Job drawing, mm, ordinate dimensions from the low corner. One solid piece. A direction names the side the tool comes from. Coordinates: 2 decimals unless noted, no trailing zeros. Loops run counter-clockwise (first coordinate to the right, second up) from the corner with the lowest first, then second, coordinate; pieces in that order, holes last. Notation, with made-up numbers: (53, 86) -> (78, 86) arc R6 cw to (78, 91) -> close; hole circle Ø4 at (39, 34). An arc over 180 degrees is marked (long way). Answer as CSV lines item,"result". Start each with the question number.
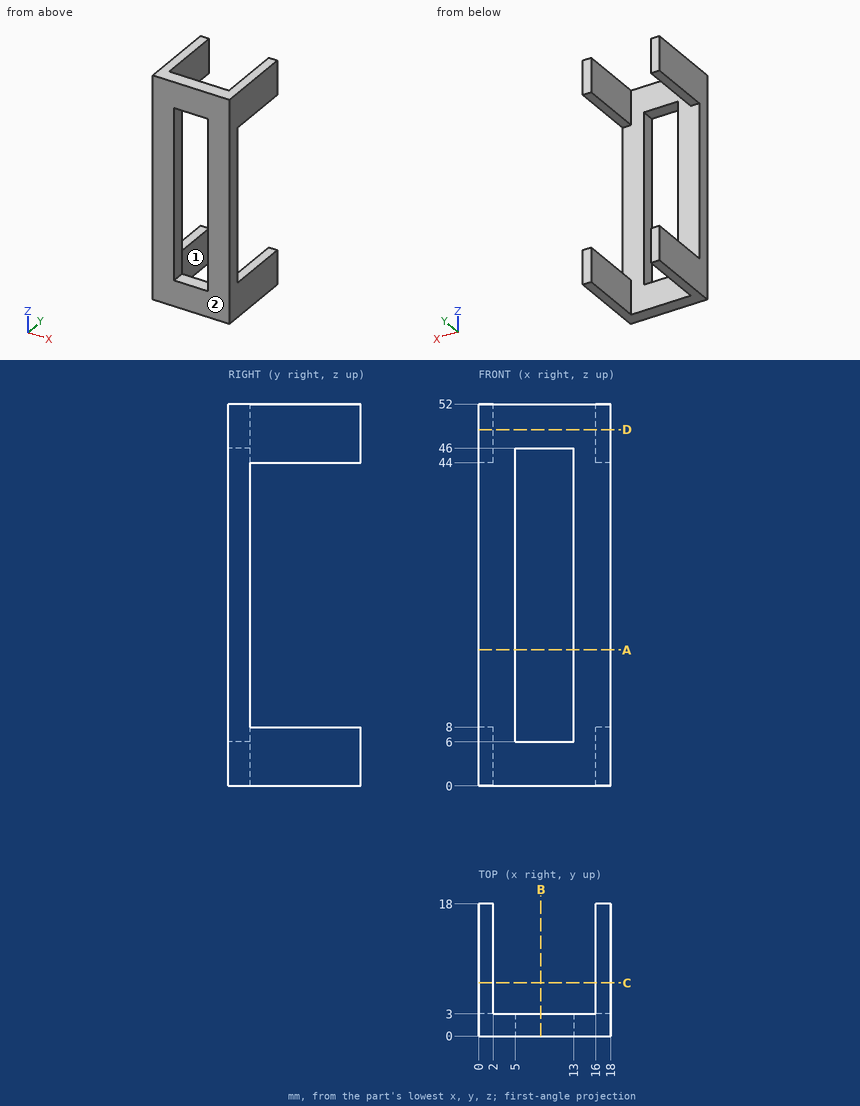
Item 1: Flat gauge pin, fed straight in: pin 1 Ø1.5 at (x, z) = (13.5, 29) entering from +Y. Where does the tip first touch, or does it go through?
Item 2: Which spindle directions (+Z, -Z, +X, -X, +Y, -Y) get a long thin tool onto all of the face, cutting with end or side? Do the marked faces 1 and 2. Say none if no direction does.
Item 3: Saw through at D-D (z = 48.5). Write the cut outline in (x, y), plus the area to 3 significant figures.
Item 4: Saw through at A-A (z = 18.5). Write the cut outline in (x, y), plus the area to 3 significant figures.
Item 5: Saw through at C-C (y = 7.25). Write the cut outline in (x, z), plus the area to 3 significant figures.
Item 6: Wall check: probe 1 along Z at (x, y) = (16.75, 13.75); probe 2 along X at (y, z) = (16.75, 45); probe 3 along Y at (x, z) = (1.5, 23). Give the ranges that are in metal, low to high.
Item 7: Saw through at B-B (x = 8.5). Write the cut outline in (y, z).
Geometry check:
1,pin 1,"y = 3"
2,face 1,"+Z, -Z, +Y"
2,face 2,"+Z, -Z, +X, -X, -Y"
3,outline,"(0, 0) -> (18, 0) -> (18, 18) -> (16, 18) -> (16, 3) -> (2, 3) -> (2, 18) -> (0, 18) -> close"
3,area,"114 mm2"
4,outline,"(0, 0) -> (5, 0) -> (5, 3) -> (0, 3) -> close; (13, 0) -> (18, 0) -> (18, 3) -> (13, 3) -> close"
4,area,"30.0 mm2"
5,outline,"(0, 0) -> (2, 0) -> (2, 8) -> (0, 8) -> close; (0, 44) -> (2, 44) -> (2, 52) -> (0, 52) -> close; (16, 0) -> (18, 0) -> (18, 8) -> (16, 8) -> close; (16, 44) -> (18, 44) -> (18, 52) -> (16, 52) -> close"
5,area,"64.0 mm2"
6,probe 1,"0 to 8, 44 to 52"
6,probe 2,"0 to 2, 16 to 18"
6,probe 3,"0 to 3"
7,outline,"(0, 0) -> (3, 0) -> (3, 6) -> (0, 6) -> close; (0, 46) -> (3, 46) -> (3, 52) -> (0, 52) -> close"
